Input: dimensioned drawing with shaded views. Units: mm. Origin: part minimum x, y, z. Round coordinates to 2 decimals unless told otherwise and drop trailing zeros. Loops run counter-clockwise (first coordinate to the right, second up) from the corner with the lowest first, then second, coordinate; pieces in that order, holes last. Notation, with made-up numbers: M 9,74 L 54,74 A13 cw 54,90 Z; hole C 20.25,84 d2. An arc over 180 degrees is marked long. Answer as a JSON object with one key per item and string values.
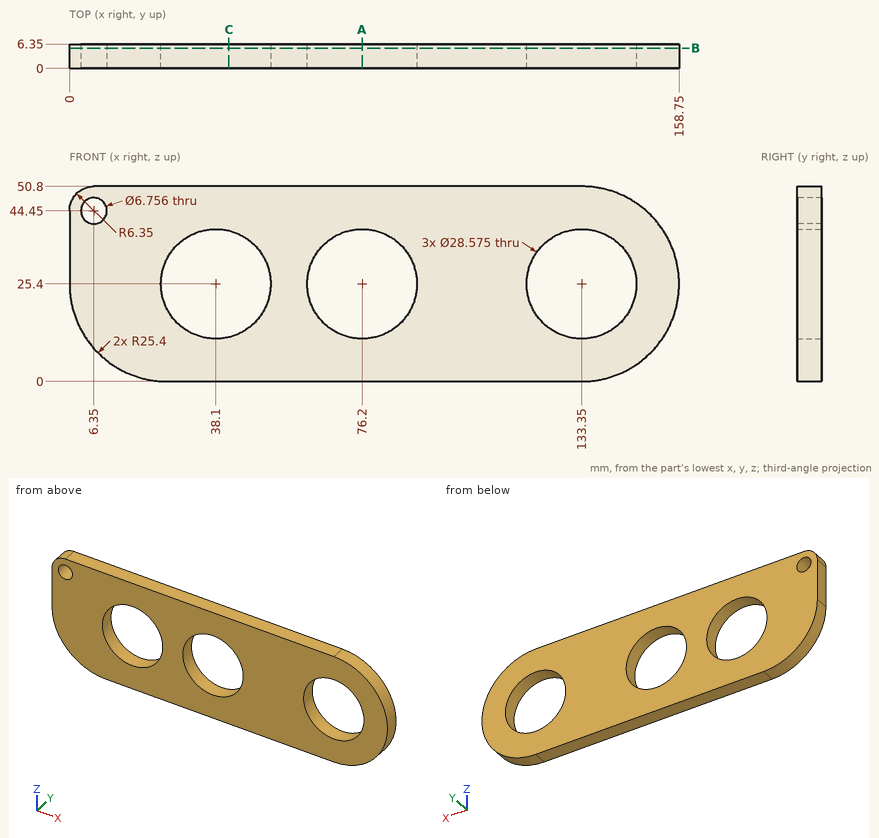
Item 1: Section A-A on x = 76.2. Return the cut outline in (y, z), then the cut area to 3 significant figures.
Answer sheet:
{"outline": "M 0,0 L 6.35,0 L 6.35,11.11 L 0,11.11 Z; M 0,39.69 L 6.35,39.69 L 6.35,50.8 L 0,50.8 Z", "area": "141 mm²"}
Item 2: Section B-B on y = 5.25. Give the number of separate pieces and of enclosed holes in the cut face, then the cut area to 3 significant figures.
Answer sheet:
{"separate pieces": "1", "enclosed holes": "4", "area": "5,680 mm²"}
Item 3: Contact query for flat-ended pins moving along their axis: pin 1 Ø2 at (y, z) = (5, 12.5) entering from -X; pin 2 Ø1.5 at (y, z) = (1.5, 32) entering from +X. Output: stop coordinate, or through.
Answer sheet:
{"pin 1": "stops at x = 2.96", "pin 2": "stops at x = 158.07"}
Item 4: Section C-C on x = 41.5. Return the cut outline in (y, z).
Answer sheet:
{"outline": "M 0,0 L 6.35,0 L 6.35,11.52 L 0,11.52 Z; M 0,39.28 L 6.35,39.28 L 6.35,50.8 L 0,50.8 Z"}
Item 5: Line query: probe 1 along X at (y, z) = (6, 24.5); probe 2 along Z at (x, y) = (38.1, 1.5); probe 3 along X at (y, z) = (0.75, 23) (1 decimal). Output: solid intervals per line, ascending. Write a range as from..to.
Answer sheet:
{"probe 1": "x = 0.02..23.84, 52.36..61.94, 90.46..119.09, 147.61..158.73", "probe 2": "z = 0..11.11, 39.69..50.8", "probe 3": "x = 0.1..24, 52.2..62.1, 90.3..119.3, 147.4..158.6"}
